```python
from build123d import *

# Parameters (mm, degrees)
BOSS_EXTRUDE1_DEPTH = 3.25
SKETCH2_W           = 25.25
SKETCH2_H           = 13
CUT_EXTRUDE1_DEPTH  = 1.5
FILLET1_R           = 2
CHAMFER1_SIZE       = 0.4


with BuildPart() as part:
    # Sketch1 → Boss-Extrude1 (new body, symmetric)
    with BuildSketch(Plane(origin=(0, 0, 0), x_dir=(1, 0, 0), z_dir=(0, 1, 0))):
        with BuildLine():
            Line((18, 6.5), (9.797958971, 6.5))
            ThreePointArc((9.797958971, 6.5), (0, 2.5), (-9.797958971, 6.5))
            Line((-9.797958971, 6.5), (-18, 6.5))
            ThreePointArc((-18, 6.5), (-18.707106781, 6.207106781), (-19, 5.5))
            Line((-19, 5.5), (-19, -5.5))
            ThreePointArc((-19, -5.5), (-18.707106781, -6.207106781), (-18, -6.5))
            Line((-18, -6.5), (-9.797958971, -6.5))
            ThreePointArc((-9.797958971, -6.5), (0, -2.5), (9.797958971, -6.5))
            Line((9.797958971, -6.5), (18, -6.5))
            ThreePointArc((18, -6.5), (18.707106781, -6.207106781), (19, -5.5))
            Line((19, -5.5), (19, 5.5))
            ThreePointArc((19, 5.5), (18.707106781, 6.207106781), (18, 6.5))
        make_face()
        with BuildLine():
            Line((-16.75, -5.25), (-14.5, -5.25))
            ThreePointArc((-14.5, -5.25), (-14.323223305, -5.176776695), (-14.25, -5))
            Line((-14.25, -5), (-14.25, 5))
            ThreePointArc((-14.25, 5), (-14.323223305, 5.176776695), (-14.5, 5.25))
            Line((-14.5, 5.25), (-16.75, 5.25))
            ThreePointArc((-16.75, 5.25), (-16.926776695, 5.176776695), (-17, 5))
            Line((-17, 5), (-17, -5))
            ThreePointArc((-17, -5), (-16.926776695, -5.176776695), (-16.75, -5.25))
        make_face(mode=Mode.SUBTRACT)
    extrude(amount=BOSS_EXTRUDE1_DEPTH, both=True)

    # Sketch2 → Cut-Extrude1 (cut)
    with BuildSketch(Plane(origin=(0, 3.25, 0), x_dir=(1, 0, 0), z_dir=(0, 1, 0))):
        with Locations((0.375, 0)):
            Rectangle(SKETCH2_W, SKETCH2_H)
    extrude(amount=-CUT_EXTRUDE1_DEPTH, mode=Mode.SUBTRACT)

    # Fillet1
    fillet1_edges = [part.edges().sort_by_distance(p)[0] for p in [
        (9.797958971, -0.75, 6.5),
        (-9.797958971, -0.75, 6.5),
        (-9.797958971, -0.75, -6.5),
        (9.797958971, -0.75, -6.5),
    ]]
    fillet(fillet1_edges, radius=FILLET1_R)

    # Chamfer1
    chamfer1_edges = [part.edges().sort_by_distance(p)[0] for p in [
        (-9.875898463, 1.75, -6.370828693),
        (19, -3.25, 0),
        (18.707106781, -3.25, 6.207106781),
        (-14.291502622, -3.25, 6.5),
        (-18.707106781, -3.25, 6.207106781),
        (-19, -3.25, 0),
        (-18.707106781, -3.25, -6.207106781),
        (14.291502622, -3.25, -6.5),
        (18.707106781, -3.25, -6.207106781),
        (-18.707106781, 3.25, -6.207106781),
        (-19, 3.25, 0),
        (-18.707106781, 3.25, 6.207106781),
        (-15.125, 3.25, 6.5),
        (-16.926776695, -3.25, 5.176776695),
        (-15.625, -3.25, 5.25),
        (-14.323223305, -3.25, 5.176776695),
        (-14.25, -3.25, 0),
        (-14.323223305, -3.25, -5.176776695),
        (-15.625, -3.25, -5.25),
        (-16.926776695, -3.25, -5.176776695),
        (-17, -3.25, 0),
        (-16.926776695, 3.25, 5.176776695),
        (-15.625, 3.25, 5.25),
        (-14.323223305, 3.25, 5.176776695),
        (-14.25, 3.25, 0),
        (-14.323223305, 3.25, -5.176776695),
        (-15.625, 3.25, -5.25),
        (-16.926776695, 3.25, -5.176776695),
        (-17, 3.25, 0),
        (18.707106781, 3.25, 6.207106781),
        (19, 3.25, 0),
        (18.707106781, 3.25, -6.207106781),
        (15.5, 3.25, 6.5),
        (11.791502622, 1.75, 6.5),
        (-15.125, 3.25, -6.5),
        (11.791502622, 1.75, -6.5),
        (-12.25, 2.5, -6.5),
        (-11.416502622, 1.75, 6.5),
        (13, 2.5, 6.5),
        (-12.25, 3.25, 0),
        (13, 3.25, 0),
        (13, 1.75, 0),
        (13, 2.5, -6.5),
        (-12.25, 1.75, 0),
        (-12.25, 2.5, 6.5),
        (15.5, 3.25, -6.5),
        (-11.416502622, 1.75, -6.5),
        (-14.291502622, -3.25, -6.5),
        (14.291502622, -3.25, 6.5),
        (0, -3.25, 2.5),
        (0, -3.25, -2.5),
        (-9.875898463, -3.25, 6.370828693),
        (9.875898463, -3.25, 6.370828693),
        (9.875898463, -3.25, -6.370828693),
        (-9.875898463, -3.25, -6.370828693),
        (0, 1.75, -2.5),
        (0, 1.75, 2.5),
        (-9.875898463, 1.75, 6.370828693),
        (9.875898463, 1.75, 6.370828693),
        (9.875898463, 1.75, -6.370828693),
    ]]
    chamfer(chamfer1_edges, length=CHAMFER1_SIZE)


solid = part.part
```
The listing builds one solid part. Answer for the finished solid, in the listing's coordinates (mm). A direction names the side the tool comes from. Give positions to 0.01 mm unless a question says otherwise; leave off trailing zeros. Loops run counter-clockwise (first coordinate to the right, second up) from the corner with the lowest first, then second, coordinate; pieces in that order, holes last. Notation, with made-up numbers: M -29,34 L 17,34 A19 ccw 17,49 Z; hole C 14,47 d10. An arc over 180 degrees is marked long. One line per item, written item: value.
1. Find the intervals of material crossed by probe 1 along X at (y, z) = (2.25, -2.75); probe 2 along X at (y, z) = (-1.5, -2); probe 3 along Z at (x, y) = (-15, -1.75), in increasing order.
Found:
probe 1: -19 to -17, -14.25 to -12.25, 13 to 19
probe 2: -19 to -17, -14.25 to 19
probe 3: -6.5 to -5.25, 5.25 to 6.5
2. Section B-B on z = -0.5 is taken. Determine the outline of the cut face in (x, y).
Found:
outline: M -19,-2.85 L -18.6,-3.25 L -17.4,-3.25 L -17,-2.85 L -17,2.85 L -17.4,3.25 L -18.6,3.25 L -19,2.85 Z; M -14.25,-2.85 L -13.85,-3.25 L 18.6,-3.25 L 19,-2.85 L 19,2.85 L 18.6,3.25 L 13.4,3.25 L 13,2.85 L 13,2.15 L 12.6,1.75 L -11.85,1.75 L -12.25,2.15 L -12.25,2.85 L -12.65,3.25 L -13.85,3.25 L -14.25,2.85 Z
3. Section D-D on z = 3.5 is taken. State how many separate pieces and enclosed holes the cut face has, plus the area to 3 significant figures.
Found:
separate pieces: 3
enclosed holes: 0
area: 138 mm^2
4. For a pull along X with two mould halves and no side action, classify faces 1 (the face through (14, 0, -6.5)), 2 (the face through (0.1, -0.7, -2.5)), 3 (the face through (-18.542, -3.092, 6.03)) as pulls with the +X half, pulls with the -X half, needs draft (parallel to the pull), parting line crosses it, or undercut.
Found:
face 1: needs draft
face 2: undercut
face 3: pulls with the -X half
5. Section A-A on y = -1 is taken. Determine the outline of the cut face in (x, z), plus the area to 3 significant figures.
Found:
outline: M -19,-5.5 A1 ccw -18,-6.5 L -10.58,-6.5 A2 ccw -9.26,-6 A14 cw 9.26,-6 A2 ccw 10.58,-6.5 L 18,-6.5 A1 ccw 19,-5.5 L 19,5.5 A1 ccw 18,6.5 L 10.58,6.5 A2 ccw 9.26,6 A14 cw -9.26,6 A2 ccw -10.58,6.5 L -18,6.5 A1 ccw -19,5.5 Z; hole M -17,-5 A0.25 ccw -16.75,-5.25 L -14.5,-5.25 A0.25 ccw -14.25,-5 L -14.25,5 A0.25 ccw -14.5,5.25 L -16.75,5.25 A0.25 ccw -17,5 Z
area: 356 mm^2
6. For faces 4 (the face through (12.926, 1.835, -6.342)), 5 (the face through (9.885, -0.779, 6.374)), 6 (the face through (19, 0, 0)), 7 (the face through (9.885, -0.721, -6.374)), determine the directions among +Z, -Z, +X, -X, +Y, -Y from which every point of the face is accessible in a straight line to the end or side of a thin tool.
Found:
face 4: -Z, +Y
face 5: +Z, +Y, -Y
face 6: +Z, -Z, +X, +Y, -Y
face 7: -Z, +Y, -Y
7. Section C-C on x = 12 is taken. Determine the outline of the cut face in (y, z), plus the area to 3 significant figures.
Found:
outline: M -3.25,-6.1 L -2.85,-6.5 L 1.35,-6.5 L 1.75,-6.1 L 1.75,6.1 L 1.35,6.5 L -2.85,6.5 L -3.25,6.1 Z
area: 64.7 mm^2
8. Each of these flat-tipped pins is pushed along its axis until it touches: P1, Ø5, axis at x = 6, z = -1.5, coming from the +Y side; P2, Ø1.5, axis at x = 2, y = 0, coming from the -Z side; P3, Ø2, axis at x = -7.5, y = -2, coming from the -Z side; P4, Ø3, axis at x = 10.5, y = 2.5, coming from the +Z side. Where does it stop, or does it pass through?
Found:
P1: y = 1.75
P2: z = -2.77
P3: z = -5.38
P4: z = 6.5
